Geometry check sheet. Reference: the model listing, model coordinates, mm. Face numbers are marked on the shaded views. A direction names the side the tool comes from. Round coordinates to 2 decimals unless told otherwise and drop trailing zeros. Order: outer loops, then holes, each group sorted by start corner. A loop starts at its lowest first (then second) coordinate and runs counter-clockwise, first axis right, second up. Notation, with made-up numbers: M 31,47.25 L 62,47.25 A6 ccw 62,56.25 Z; hole C 57,25 d5. An arc over 180 degrees is marked long. Answer as a JSON object with one key per item and string values. Group by question number.
```python
from build123d import *

# Parameters (mm, degrees)
FILLET_R     = 0.5
CHAMFER_SIZE = 0.4


with BuildPart() as part:
    # Sketch → Revolution (revolve)
    with BuildSketch(Plane.XZ):
        Polygon((2.25, 0), (2.25, 2.5), (8.557962, 2.5), (8.557962, 0), (7.5, -6), (4.25, -6), (4.25, 0), align=None)
    revolve(axis=Axis((0, 0, 0), (0, 0, 1)))

    # Fillet
    fillet_edges = [part.edges().sort_by_distance(p)[0] for p in [
        (-7.5, 0, -6),
        (-4.25, 0, -6),
    ]]
    fillet(fillet_edges, radius=FILLET_R)

    # Chamfer
    chamfer_edges = [part.edges().sort_by_distance(p)[0] for p in [
        (-2.25, 0, 2.5),
        (-8.557962, 0, 2.5),
    ]]
    chamfer(chamfer_edges, length=CHAMFER_SIZE)


solid = part.part
```
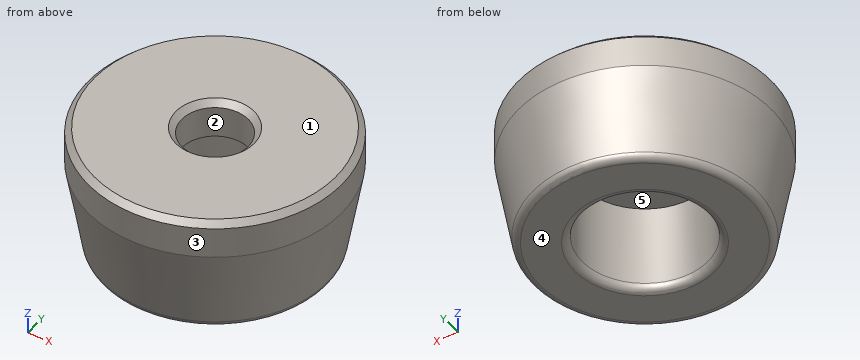
1) Go/stop test with flat-tipped pins: P1, Ø1.5, axis at y = -2, z = -1.5, coming from the +X side; P2, Ø7, axis at x = 1.5, y = -1.5, coming from the -Z side; P3, Ø3, axis at x = -3.5, z = -1.5, coming from the -Y side. Record where each tip stops, or that it passes through.
2) Set-up check for the marked faces 4 and 5: record each of +Z, -Z, +X, -X, +Y, -Y from which the full face is reachable in a straight line by a thin tool's end or side.
3) Sectioned sample at D-D (z = -3). Record the boundary of the cut face in (x, y).
4) Sectioned sample at A-A (y = 0). Record the boundary of the cut face in (x, z).
5) Release check for a two-part mould opening along Y. For the marked faces 1, 2 and 3 record: +Y half, -Y half, draft (parallel to the pull), parting line (faces both ways), or undercut.
6) Sectioned sample at C-C (z = -1.25). Record the boundary of the cut face in (x, y), then the cut area to 3 significant figures.
7) Thickness scan on line 1 along Y through (x, z) = (0, 1.2); line 2 along X through (y, z) = (-0.5, -2); line 3 along X through (y, z) = (1.25, 0.5). Record the ranges inside material, lowest first. Write a range as [from, to].
Final values:
{
 "1": {"P1": "stops at x = 8.26", "P2": "stops at z = -6", "P3": "stops at y = -8.13"},
 "2": {"face 4": "-Z, +X, -X, +Y, -Y", "face 5": "-Z"},
 "3": {"outline": "C 0,0 d16.06; hole C 0,0 d8.5"},
 "4": {"outline": "M -8.56,0 L -7.57,-5.59 A0.5 ccw -7.08,-6 L -4.75,-6 A0.5 ccw -4.25,-5.5 L -4.25,0 L -2.25,0 L -2.25,2.1 L -2.65,2.5 L -8.16,2.5 L -8.56,2.1 Z; M 2.25,0 L 4.25,0 L 4.25,-5.5 A0.5 ccw 4.75,-6 L 7.08,-6 A0.5 ccw 7.57,-5.59 L 8.56,0 L 8.56,2.1 L 8.16,2.5 L 2.65,2.5 L 2.25,2.1 Z"},
 "5": {"face 1": "draft", "face 2": "undercut", "face 3": "parting line"},
 "6": {"outline": "C 0,0 d16.68; hole C 0,0 d8.5", "area": "162 mm^2"},
 "7": {"line 1": "y = [-8.56, -2.25], [2.25, 8.56]", "line 2": "x = [-8.19, -4.22], [4.22, 8.19]", "line 3": "x = [-8.47, -1.87], [1.87, 8.47]"}
}
